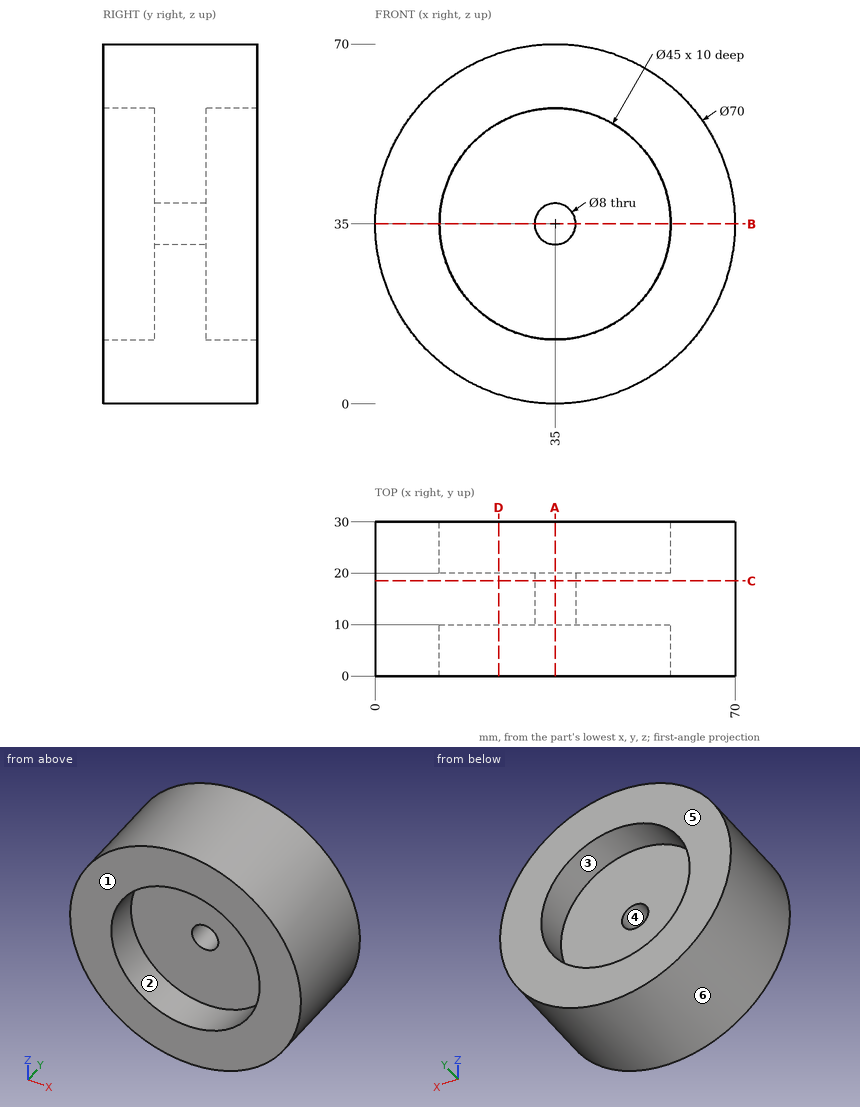
Here's the drawing with two shaded views (mm, measured from the low corner). I have some questions. A direction names the side the tool comes from. Coordinates: 2 decimals unless noted, no trailing zeros. Order: outer loops, then holes, each group sorted by start corner. A loop starts at its lowest first (then second) coordinate and runs counter-clockwise, first axis right, second up. Notation, with made-up numbers: M 57,66.25 L 84,66.25 A25 ccw 84,98.25 Z; hole C 82.25,56 d8. An arc over 180 degrees is marked long. Write item = value, one per line.
(1) For pin 1 Ø8 at (x, z) = (43.5, 22.5) entering from +Y; pin 2 Ø13.5 at (x, z) = (37.5, 46) entering from -Y; pin 3 Ø1.5 at (x, y) = (11, 14) entering from -Z, each with a flat end and sliding along its axis, tell me the tip position at first contact or that it passes through.
Results are:
pin_1 = 20
pin_2 = 10
pin_3 = 8.84
(2) If we mould it in two halves opening along X, with no side actions, what happens to the marked faces 4, 5 and 6? For each: pulls with the +X half, pulls with the -X half, needs draft (parallel to the pull), parting line crosses it, or undercut.
Results are:
face_4 = undercut
face_5 = needs draft
face_6 = parting line crosses it
(3) Suppose I cut it at C-C on y = 18.5. Please give me the cut outline in (x, z).
Results are:
outline = C 35,35 d70; hole C 35,35 d8
(4) For the marked faces 1, 2 and 3, which set-ups out of +Z, -Z, +X, -X, +Y, -Y let a thin tool reach every point of the face, with its end or its side?
Results are:
face_1 = +Z, -Z, +X, -X, -Y
face_2 = -Y
face_3 = +Y
(5) I need wall thicknesses on line 1 along X through (y, z) = (25, 35); line 2 along X through (y, z) = (13.5, 35); line 3 along Z through (x, y) = (37, 12). Which ranges of each line are inside material? Lowest first, please. Write a range as [from, to].
Results are:
line_1 = [0, 12.5], [57.5, 70]
line_2 = [0, 31], [39, 70]
line_3 = [0.06, 31.54], [38.46, 69.94]
(6) Suppose I cut it at A-A on x = 35. Please give me the cut outline in (y, z), plus the area to 3 significant figures.
Results are:
outline = M 0,0 L 30,0 L 30,12.5 L 20,12.5 L 20,31 L 10,31 L 10,12.5 L 0,12.5 Z; M 0,57.5 L 10,57.5 L 10,39 L 20,39 L 20,57.5 L 30,57.5 L 30,70 L 0,70 Z
area = 1,120 mm2
(7) Suppose I cut it at B-B on z = 35. Please give me the cut outline in (x, y).
Results are:
outline = M 0,0 L 12.5,0 L 12.5,10 L 31,10 L 31,20 L 12.5,20 L 12.5,30 L 0,30 Z; M 39,10 L 57.5,10 L 57.5,0 L 70,0 L 70,30 L 57.5,30 L 57.5,20 L 39,20 Z
(8) Suppose I cut it at D-D on x = 24. Please give me the cut outline in (y, z).
Results are:
outline = M 0,1.77 L 30,1.77 L 30,15.37 L 20,15.37 L 20,54.63 L 30,54.63 L 30,68.23 L 0,68.23 L 0,54.63 L 10,54.63 L 10,15.37 L 0,15.37 Z
